```python
from build123d import *

# Parameters (mm, degrees)
F2_R     = 1.5
F3_DEPTH = 12.7
F5_DEPTH = 12.5


with BuildPart() as f1:
    # F0 (on Front) → F1 (revolve)
    with BuildSketch(Plane.XZ):
        with BuildLine():
            Line((0, 5.227802), (0, 3.5))
            Line((0, 3.5), (13.300416, 3.5))
            Line((13.300416, 3.5), (13.300416, 2))
            Line((13.300416, 2), (15, 2))
            Line((15, 2), (15, 0))
            Line((15, 0), (118, 0))
            Line((118, 0), (118, 1.055168))
            ThreePointArc((118, 1.055168), (117.12132, 3.176489), (115, 4.055168))
            Line((115, 4.055168), (100.770019, 4.055168))
            Line((100.770019, 4.055168), (95.903615, 5.61387))
            Line((95.903615, 5.61387), (92.819303, 5.61387))
            Line((92.819303, 5.61387), (92.819303, 8.060487))
            Line((92.819303, 8.060487), (82.9174, 8.060487))
            Line((82.9174, 8.060487), (82.9174, 6.148748))
            Line((82.9174, 6.148748), (81.859961, 6.148748))
            Line((81.859961, 6.148748), (81.859961, 8.060487))
            Line((81.859961, 8.060487), (79.733633, 8.060487))
            Line((79.733633, 8.060487), (79.733633, 5.61387))
            Line((79.733633, 5.61387), (76.3731, 5.61387))
            Line((76.3731, 5.61387), (76.3731, 8.060487))
            Line((76.3731, 8.060487), (74.226245, 8.060487))
            Line((74.226245, 8.060487), (74.226245, 6.098706))
            Line((74.226245, 6.098706), (72.943754, 6.098706))
            Line((72.943754, 6.098706), (72.943754, 8.060487))
            Line((72.943754, 8.060487), (70.152812, 8.060487))
            Line((70.152812, 8.060487), (70.152812, 5.870874))
            Line((70.152812, 5.870874), (66.633068, 5.870874))
            Line((66.633068, 5.870874), (66.633068, 8.060487))
            Line((66.633068, 8.060487), (64.490482, 8.060487))
            Line((64.490482, 8.060487), (64.490482, 5.859734))
            Line((64.490482, 5.859734), (63.669845, 5.859734))
            Line((63.669845, 5.859734), (63.669845, 8.060487))
            Line((63.669845, 8.060487), (61.918698, 8.060487))
            Line((61.918698, 8.060487), (61.918698, 5.5))
            Line((61.918698, 5.5), (33.415843, 5.5))
            Line((33.415843, 5.5), (33.415843, 6.582501))
            Line((33.415843, 6.582501), (30.852729, 6.582501))
            Line((30.852729, 6.582501), (30.852729, 5.927347))
            Line((30.852729, 5.927347), (29.827483, 5.927347))
            Line((29.827483, 5.927347), (29.827483, 7.679923))
            Line((29.827483, 7.679923), (27.20741, 7.679923))
            Line((27.20741, 7.679923), (27.20741, 6.861783))
            Line((27.20741, 6.861783), (26.188558, 6.861783))
            Line((26.188558, 6.861783), (25.678367, 8.63155))
            Line((25.678367, 8.63155), (21.340726, 8.63155))
            Line((21.340726, 8.63155), (21.340726, 7.579132))
            Line((21.340726, 7.579132), (18.834569, 7.579132))
            Line((18.834569, 7.579132), (18.834569, 6.582501))
            Line((18.834569, 6.582501), (17.069861, 6.582501))
            Line((17.069861, 6.582501), (17.069861, 5.295536))
            Line((17.069861, 5.295536), (7.069861, 5.295536))
            Line((7.069861, 5.295536), (5.376487, 8))
            Line((5.376487, 8), (1.989738, 8))
            Line((1.989738, 8), (1.989738, 5.227802))
            Line((1.989738, 5.227802), (0, 5.227802))
        make_face()
    revolve(axis=Axis((66.5, 0, 0), (1, 0, 0)))

    # F2 (on Front) → F3 (cut, symmetric)
    with BuildSketch(Plane.XZ):
        with Locations((112, 0)):
            Circle(F2_R)
    extrude(amount=F3_DEPTH, both=True, mode=Mode.SUBTRACT)

    # F4 (on Top) → F5 (cut, symmetric)
    with BuildSketch(Plane.XY):
        with BuildLine():
            Line((119.202645, 1.249984), (108.006297, 1.249984))
            ThreePointArc((108.006297, 1.249984), (106.750004, 0.003148), (108, -1.25))
            Line((108, -1.25), (119.202645, -1.25))
            Line((119.202645, -1.25), (119.202645, 1.249984))
        make_face()
    extrude(amount=F5_DEPTH, both=True, mode=Mode.SUBTRACT)


solid = f1.part
```
Could you check a few things on this model? Use its own coordinates, in mm. A direction names the side the tool comes from. Round coordinates to 2 decimals unless told otherwise and drop trailing zeros. Loops run counter-clockwise (first coordinate to the right, second up) from the corner with the lowest first, then second, coordinate; pieces in that order, holes last. Notation, with made-up numbers: (-9.5, 71.5) - (1.5, 71.5) arc R37 cw to (1.5, 107.5) - close; hole circle Ø4 at (23, 86.5). An arc over 180 degrees is marked (long way). Use CSV: the item, a comma, the result in double quotes.
Item 1: If we section it at D-D on x = 41: List the corners of the cut face in (y, z) for me, then the cut area to 3 significant figures.
Here are the results:
outline,"circle Ø11 at (0, 0)"
area,"95.0 mm²"
Item 2: I need wall thicknesses on L1, parallel to Y at x = 13.8, z = 0; L2, parallel to Z at x = 9.5, y = 0. Which ranges of each line are inside material? Lowest first, please. Write a range as [from, to].
Here are the results:
L1,"y = [-5.3, -2], [2, 5.3]"
L2,"z = [-5.3, -3.5], [3.5, 5.3]"
Item 3: If we mould it in two halves opening along X, with no side actions, what happens to faces 4 (the cylindrical face through (0.981, -1.57, 4.986)), 5 (the cylindrical face through (110.5, 2.63, 0.07)), 6 (the flat face through (13.3, 2, 2))? For each: pulls with the +X half, pulls with the -X half, needs draft (parallel to the pull), parting line crosses it, or undercut.
Here are the results:
face 4,"needs draft"
face 5,"undercut"
face 6,"pulls with the -X half"
Item 4: Will these pins go through, and if not, where does the flat tip stop? pin 1 (5 mm diameter, centred on x = 41, y = 4, fed in from -Z); pin 2 (5 mm diameter, centred on x = 43.5, z = 0.5, fed in from +Y); pin 3 (4 mm diameter, centred on y = 7, z = -4.5, fed in from +X).
Here are the results:
pin 1,"stops at z = -5.29"
pin 2,"stops at y = 5.5"
pin 3,"stops at x = 92.82"
Item 5: If we section it at C-C on x = 85: List the corners of the cut face in (y, z) for me.
Here are the results:
outline,"circle Ø16.12 at (0, 0)"
Item 6: If we section it at A-A on x = 112: List the corners of the cut face in (y, z) for me, then the cut area to 3 significant figures.
Here are the results:
outline,"(-3.77, -1.5) arc R4.06 ccw to (-1.25, -3.86) - (-1.25, -1.5) - close; (-3.77, 1.5) - (-1.25, 1.5) - (-1.25, 3.86) arc R4.06 ccw to start; (1.25, -3.86) arc R4.06 ccw to (3.77, -1.5) - (1.25, -1.5) - close; (1.25, 1.5) - (3.77, 1.5) arc R4.06 ccw to (1.25, 3.86) - close"
area,"15.4 mm²"
Item 7: If we section it at B-B on z = 0: Count the separate pieces of the cut face and the enclosed holes in it, then the cut area to 3 significant figures.
Here are the results:
separate pieces,"3"
enclosed holes,"0"
area,"1,290 mm²"
Item 8: For faces 1 (the cylindrical face through (3.66, 7.81, -1.73)), 2 (the flat face through (27.207, -5, -5)), 3 (the flat face through (114, 1.25, 0)), which set-ups out of +Z, -Z, +X, -X, +Y, -Y let a thin tool reach every point of the face, with its end or its side?
Here are the results:
face 1,"-X"
face 2,"none"
face 3,"+Z, -Z, +X"
